```python
from build123d import *

# Parameters (mm, degrees)
EXTRUDE_1_DEPTH     = 8
SKETCH_2_R          = 6
SKETCH_2_R_2        = 2.75
CUT_EXTRUDE_1_DEPTH = 8
SKETCH_3_R          = 2.75
CUT_EXTRUDE_2_DEPTH = 10
SKETCH_4_W          = 32.5
SKETCH_4_H          = 40
CUT_EXTRUDE_3_DEPTH = 10
FILLET_1_R          = 5
SKETCH_5_R          = 2.75
CUT_EXTRUDE_4_DEPTH = 230.869528211
SKETCH_6_W          = 20
SKETCH_6_H          = 20
CUT_EXTRUDE_5_DEPTH = 230.869528211
FILLET_2_R          = 3
SKETCH_7_R          = 1.5
SKETCH_7_R_2        = 2.75
CUT_EXTRUDE_6_DEPTH = 230.869528211
SKETCH_8_W          = 20
SKETCH_8_H          = 20
CUT_EXTRUDE_7_DEPTH = 230.869528211
FILLET_3_R          = 3


with BuildPart() as part:
    # 草图1 → 凸台-拉伸1 (new body)
    with BuildSketch(Plane(origin=(0, 0, 0), x_dir=(0, 0, -1), z_dir=(1, 0, 0))):
        with BuildLine():
            Line((-150, 100.619037897), (-150, -100.619037897))
            ThreePointArc((-150, -100.619037897), (0, -174), (150, -100.619037897))
            Line((150, -100.619037897), (150, 100.619037897))
            ThreePointArc((150, 100.619037897), (0, 174), (-150, 100.619037897))
        make_face()
    extrude(amount=EXTRUDE_1_DEPTH)

    # 草图2 → 切除-拉伸1 (cut)
    with BuildSketch(Plane(origin=(8, 0, 0), x_dir=(0, 0, -1), z_dir=(1, 0, 0))):
        with Locations((97.5, 45)):
            Circle(SKETCH_2_R)
        with Locations((97.5, -45)):
            Circle(SKETCH_2_R)
        with Locations((85.75, 52.5)):
            Circle(SKETCH_2_R_2)
        with Locations((109.25, 52.5)):
            Circle(SKETCH_2_R_2)
        with Locations((85.75, -52.5)):
            Circle(SKETCH_2_R_2)
        with Locations((109.25, -52.5)):
            Circle(SKETCH_2_R_2)
        with Locations(Location((-109.25, -52.5, 0), (0, 0, 180))):
            Circle(SKETCH_2_R_2)
        with Locations(Location((-85.75, -52.5, 0), (0, 0, 180))):
            Circle(SKETCH_2_R_2)
        with Locations(Location((-109.25, 52.5, 0), (0, 0, 180))):
            Circle(SKETCH_2_R_2)
        with Locations(Location((-85.75, 52.5, 0), (0, 0, 180))):
            Circle(SKETCH_2_R_2)
        with Locations(Location((-97.5, -45, 0), (0, 0, 180))):
            Circle(SKETCH_2_R)
        with Locations(Location((-97.5, 45, 0), (0, 0, 180))):
            Circle(SKETCH_2_R)
    extrude(amount=-CUT_EXTRUDE_1_DEPTH, mode=Mode.SUBTRACT)

    # 草图3 → 切除-拉伸2 (cut)
    with BuildSketch(Plane(origin=(8, 0, 0), x_dir=(0, 0, -1), z_dir=(1, 0, 0))):
        with Locations((-40, 60)):
            Circle(SKETCH_3_R)
        with Locations((40, 60)):
            Circle(SKETCH_3_R)
        with Locations((40, -60)):
            Circle(SKETCH_3_R)
        with Locations((-40, -60)):
            Circle(SKETCH_3_R)
        with Locations((40, 0)):
            Circle(SKETCH_3_R)
        with Locations((-40, 0)):
            Circle(SKETCH_3_R)
    extrude(amount=-CUT_EXTRUDE_2_DEPTH, mode=Mode.SUBTRACT)

    # 草图4 → 切除-拉伸3 (cut)
    with BuildSketch(Plane(origin=(8, 0, 0), x_dir=(0, 0, -1), z_dir=(1, 0, 0))):
        with Locations((133.75, 0)):
            Rectangle(SKETCH_4_W, SKETCH_4_H)
        with Locations((-133.75, 0)):
            Rectangle(SKETCH_4_W, SKETCH_4_H)
    extrude(amount=-CUT_EXTRUDE_3_DEPTH, mode=Mode.SUBTRACT)

    # 圆角1
    fillet_1_edges = [part.edges().sort_by_distance(p)[0] for p in [
        (4, -20, -117.5),
        (4, 20, -117.5),
        (4, 20, -150),
        (4, -20, -150),
        (4, 20, 150),
        (4, 20, 117.5),
        (4, -20, 117.5),
        (4, -20, 150),
    ]]
    fillet(fillet_1_edges, radius=FILLET_1_R)

    # 草图5 → 切除-拉伸4 (cut, through all)
    with BuildSketch(Plane(origin=(8, 0, 0), x_dir=(0, 0, -1), z_dir=(1, 0, 0))):
        with Locations((50, 150)):
            Circle(SKETCH_5_R)
        with Locations((-50, 150)):
            Circle(SKETCH_5_R)
        with Locations((-50, 120)):
            Circle(SKETCH_5_R)
        with Locations((50, 120)):
            Circle(SKETCH_5_R)
    extrude(amount=-CUT_EXTRUDE_4_DEPTH, mode=Mode.SUBTRACT)

    # 草图6 → 切除-拉伸5 (cut, through all)
    with BuildSketch(Plane(origin=(8, 0, 0), x_dir=(0, 0, -1), z_dir=(1, 0, 0))):
        with Locations((-90, 90)):
            Rectangle(SKETCH_6_W, SKETCH_6_H)
        with Locations((90, 90)):
            Rectangle(SKETCH_6_W, SKETCH_6_H)
    extrude(amount=-CUT_EXTRUDE_5_DEPTH, mode=Mode.SUBTRACT)

    # 圆角2
    fillet_2_edges = [part.edges().sort_by_distance(p)[0] for p in [
        (4, 80, 100),
        (4, 100, 100),
        (4, 100, 80),
        (4, 80, 80),
        (4, 100, -80),
        (4, 100, -100),
        (4, 80, -100),
        (4, 80, -80),
    ]]
    fillet(fillet_2_edges, radius=FILLET_2_R)

    # 草图7 → 切除-拉伸6 (cut, through all)
    with BuildSketch(Plane(origin=(8, 0, 0), x_dir=(0, 0, -1), z_dir=(1, 0, 0))):
        with Locations((-30, -105)):
            Circle(SKETCH_7_R)
        with Locations((-30, -145)):
            Circle(SKETCH_7_R)
        with Locations((30, -145)):
            Circle(SKETCH_7_R)
        with Locations((30, -105)):
            Circle(SKETCH_7_R)
        with Locations((120, -100)):
            Circle(SKETCH_7_R_2)
        with Locations((100, -130)):
            Circle(SKETCH_7_R_2)
        with Locations(Location((-100, -130, 0), (0, 0, 180))):
            Circle(SKETCH_7_R_2)
        with Locations(Location((-120, -100, 0), (0, 0, 180))):
            Circle(SKETCH_7_R_2)
    extrude(amount=-CUT_EXTRUDE_6_DEPTH, mode=Mode.SUBTRACT)

    # 草图8 → 切除-拉伸7 (cut, through all)
    with BuildSketch(Plane(origin=(8, 0, 0), x_dir=(0, 0, -1), z_dir=(1, 0, 0))):
        with Locations((60, -135)):
            Rectangle(SKETCH_8_W, SKETCH_8_H)
        with Locations((-60, -135)):
            Rectangle(SKETCH_8_W, SKETCH_8_H)
    extrude(amount=-CUT_EXTRUDE_7_DEPTH, mode=Mode.SUBTRACT)

    # 圆角3
    fillet_3_edges = [part.edges().sort_by_distance(p)[0] for p in [
        (4, -145, -50),
        (4, -125, -50),
        (4, -125, -70),
        (4, -145, -70),
        (4, -125, 70),
        (4, -125, 50),
        (4, -145, 50),
        (4, -145, 70),
    ]]
    fillet(fillet_3_edges, radius=FILLET_3_R)


solid = part.part
```
Source: CAD feature listing. Evaluate the final solid. Frame: model axes, mm. A direction names the side the tool comes from. Coordinates: 2 decimals unless noted, no trailing zeros. Loops run counter-clockwise (first coordinate to the right, second up) from the corner with the lowest first, then second, coordinate; pieces in that order, holes last. Notation, with made-up numbers: (-38.5, -33) -> (17.5, -33) arc R22 ccw to (17.5, 6) -> close; hole circle Ø2 at (-37.75, -19.5). An arc over 180 degrees is marked (long way). One line per item, written item: value. Start each with the question number.
Q1. Contact query for flat-ended pins moving along their axis: P1, Ø2, axis at y = -2.5, z = 48.5, coming from the -X side; P2, Ø3, axis at x = 5, y = -130.5, coming from the +Z side; P3, Ø1, axis at x = 4.5, z = 67, coming from the -Y side; P4, Ø2.5, axis at x = 5.5, y = -5.5, coming from the +Z side. Output: stop coordinate, or through.
Q2. Line query: line 1 along Z through (x, y) = (4.5, 92); line 2 along Z through (x, y) = (6, -52); line 3 along Y through (x, z) = (2.25, 97.5). Output: solid intervals per line, ascending.
Q3. Mould query, pull axis Y, two halves, no side actions, for faces 4 (the face through (4, 90, -80)), 5 (the face through (3.944, 173.985, -2.42)), 6 (the face through (4, 63, 150)), 7 (the face through (4, -20, 134)). Classes: pulls with the +Y half, pulls with the -Y half, needs draft (parallel to the pull), parting line crosses it, or undercut.
Q4. Set-up query: faces 1 (the face through (4, 0, 117.5)), 2 (the face through (4, -135, 70)), 3 (the face through (4, 0, -117.5)). Return all of +Z, -Z, +X, -X, +Y, -Y with unobstructed straight access to the full face (end or side cutting, diameter ignored); none if empty.
Q5. Section query A-A, the plane x = 3.25. Give the number of separate pieces and of enclosed holes in the cut face, and give its area (3 significant figures).
Q6. Section query B-B, the plane y = -111.5. Return the cut outline in (x, z).
Results:
1. P1: x = 0
1. P2: z = 122.78
1. P3: y = -161.98
1. P4: z = 117.5
2. line 1: -150 to -100, -80 to 80, 100 to 150
2. line 2: -150 to -111.95, -106.55 to -88.45, -83.05 to 83.05, 88.45 to 106.55, 111.95 to 150
2. line 3: -147.08 to -131.15, -128.85 to -51, -39 to 39, 51 to 80.04, 99.96 to 147.08
3. face 4: undercut
3. face 5: pulls with the +Y half
3. face 6: needs draft
3. face 7: undercut
4. face 1: +Z, +X, -X
4. face 2: +X, -X
4. face 3: -Z, +X, -X
5. separate pieces: 1
5. enclosed holes: 34
5. area: 85,900 mm^2
6. outline: (0, -140.87) -> (8, -140.87) -> (8, 140.87) -> (0, 140.87) -> close
